```python
from build123d import *

# Parameters (mm, degrees)
SKETCH6_W          = 10
SKETCH6_H          = 3
SKETCH8_R          = 1.875
CUT_EXTRUDE2_DEPTH = 112.050664113
FILLET1_R          = 5


with BuildPart() as part:
    # Sweep1: sweep along a path in Sketch7
    with BuildLine(Plane(origin=(0, 0, 0), x_dir=(0, 0, -1), z_dir=(1, 0, 0))) as sweep1_path:
        Line((-1.5, 0), (-1.5, 10))
        ThreePointArc((-1.5, 10), (-1.766933397, 11.611856238), (-2.539232213, 13.051609172))
        Line((-2.539232213, 13.051609172), (-8.960767787, 21.386297467))
        ThreePointArc((-8.960767787, 21.386297467), (-9.733066603, 22.8260504), (-10, 24.437906639))
        Line((-10, 24.437906639), (-10, 55))
    # Sketch6 → Sweep1 (sweep)
    with BuildSketch(Plane(origin=(0, 0, 0), x_dir=(1, 0, 0), z_dir=(0, 1, 0))):
        with Locations((5, -1.5)):
            Rectangle(SKETCH6_W, SKETCH6_H)
    sweep(path=sweep1_path.line)

    # Mirror2: part across plane


with BuildPart() as part_1:
    add(part.part)
    add(part.part.mirror(Plane(origin=(0, 55, 8.5), x_dir=(0, 0, 1), z_dir=(0, 1, 0))))

    # Sketch8 → Cut-Extrude2 (cut, through all)
    with BuildSketch(Plane(origin=(0, 0, 0), x_dir=(-1, 0, 0), z_dir=(0, 0, -1))):
        with Locations((-5, 5)):
            Circle(SKETCH8_R)
        with Locations((-5, 105)):
            Circle(SKETCH8_R)
    extrude(amount=-CUT_EXTRUDE2_DEPTH, mode=Mode.SUBTRACT)

    # Fillet1
    fillet1_edges = [part_1.edges().sort_by_distance(p)[0] for p in [
        (0, 0, 1.5),
        (10, 0, 1.5),
        (10, 110, 1.5),
        (0, 110, 1.5),
    ]]
    fillet(fillet1_edges, radius=FILLET1_R - 0.0001)  # a hair under: the kernel refuses the full size


solid = part_1.part
```
Here's how the part is built. I have some questions about the finished solid (model axes, mm). A direction names the side the tool comes from. Give positions to 0.01 mm unless a question says otherwise; leave off trailing zeros. Write each loop counter-clockwise with the first axis right and the second up, starting at its lowest first coordinate (ties: lowest second). Pieces come first, ordered by that corner, then holes. Notation, with made-up numbers: (-34.5, 79) -> (-16.5, 79) arc R23 cw to (-16.5, 88) -> close; hole circle Ø1 at (23.5, 2). An arc over 180 degrees is marked (long way). Use one line per item in the form item = value.
1) We'd pull the mould along X, two halves only. Please class faces 4 (the face through (6.38, 6.27, 1.48)), 5 (the face through (1, 108, 2)), 6 (the face through (4.93, 93.64, 6.98)), 7 (the face through (10, 55, 9)): +X half, -X half, draft (parallel to the pull), parting line (faces both ways), or undercut.
Verdict:
face_4 = undercut
face_5 = -X half
face_6 = draft
face_7 = +X half
2) I'm going to push flat-ended pins straight in: pin 1 (3 mm diameter, centred on y = 37, z = 6.5, fed in from +X); pin 2 (4 mm diameter, centred on x = 2, y = 98, fed in from +Z); pin 3 (4 mm diameter, centred on x = 7.5, y = 97.5, fed in from +Z); pin 4 (6 mm diameter, centred on x = 2.5, y = 76, fed in from -Z). Where does each tip first touch, or does it pass through?
Verdict:
pin_1 = through
pin_2 = 5.16
pin_3 = 5.55
pin_4 = 8.5
3) Suppose I cut it at A-A (z = 6). Please give me the cut outline in (x, y).
Verdict:
outline = (0, 15.09) -> (10, 15.09) -> (10, 20) -> (0, 20) -> close; (0, 90) -> (10, 90) -> (10, 94.91) -> (0, 94.91) -> close
4) If I drill on L1, parallel to X at y = 105, z = 1.35 (3 decimals); L2, parallel to Y at x = 5, z = 1 (3 decimals); L3, parallel to Z at x = 9, y = 102.5, over which ranges is the centre line in solid material (lowest first)? Write a range as [from, to].
Verdict:
L1 = [0, 3.125], [6.875, 10]
L2 = [0, 3.125], [6.875, 13.464], [96.536, 103.125], [106.875, 110]
L3 = [0, 3]
5) On a 3-axis mill with a long thin cutter (end or side, diameter ignored), from which of +Z, -Z, +X, -X, +Y, -Y can I reach the whole of each face in a straight line? I mean faces 1 (the face through (5.1, 7.3, 0)), 2 (the face through (4.9, 7.3, 3)), 3 (the face through (5, 55, 8.5)). Say none if no direction works.
Verdict:
face_1 = -Z, +X, -X, +Y, -Y
face_2 = +Z, +X, -X, -Y
face_3 = -Z, +X, -X
6) Suppose I cut it at C-C (y = 90.5). Please give me the cut outline in (x, z).
Verdict:
outline = (0, 5.61) -> (10, 5.61) -> (10, 9.4) -> (0, 9.4) -> close
7) Suppose I cut it at D-D (y = 47.5). Please give me the cut outline in (x, z).
Verdict:
outline = (0, 8.5) -> (10, 8.5) -> (10, 11.5) -> (0, 11.5) -> close
8) Suppose I cut it at B-B (x = 1.5). Please give me the cut outline in (y, z), and give its area (3 significant figures).
Verdict:
outline = (1.43, 0) -> (10, 0) arc R6.5 ccw to (13.97, 1.35) -> (22.3, 7.77) arc R3.5 cw to (24.44, 8.5) -> (85.56, 8.5) arc R3.5 cw to (87.7, 7.77) -> (96.03, 1.35) arc R6.5 ccw to (100, 0) -> (108.57, 0) -> (108.57, 3) -> (100, 3) arc R3.5 cw to (97.86, 3.73) -> (89.53, 10.15) arc R6.5 ccw to (85.56, 11.5) -> (24.44, 11.5) arc R6.5 ccw to (20.47, 10.15) -> (12.14, 3.73) arc R3.5 cw to (10, 3) -> (1.43, 3) -> close
area = 337 mm2
